Job drawing, mm, ordinate dimensions from the low corner. One solid piece. Coordinates: 2 decimals unless noted, no trailing zeros. Loops run counter-clockwise (first coordinate to the right, second up) from the corner with the lowest first, then second, coordinate; pieces in that order, holes last. Notation, with made-up numbers: (-37.75, -19) - (-27.75, -19) arc R23 cw to (-27.75, 18) - close; hole circle Ø1 at (32.25, -25.75). An arc over 180 degrees is marked (long way). Use a Markdown table: item, result. Add a question column.
1. Wall check: probe 1 along Y at (x, z) = (6.75, 352.7); probe 2 along Z at (x, y) = (18.25, 10); probe 3 along Z at (x, y) = (1.5, 14.25). Give the ranges that are in metal, low to high. Write a range as [from, to].
2. Drop flat-ended pins along their axis: pin 1 (1.5 mm diameter, centred on y = 4, z = 226, fed in from -X); pin 2 (4 mm diameter, centred on y = 12.7, z = 352.7, fed in from -X). Give the stop position or say it passes through.
3. Band-saw the part on B-B, the plane z = 352.7. Give the cut face in (x, y), plus the area to 3 significant figures.
4. Band-saw the part on A-A, the plane y = 12.7. Give the cut face in (x, z), plus the area to 3 significant figures.
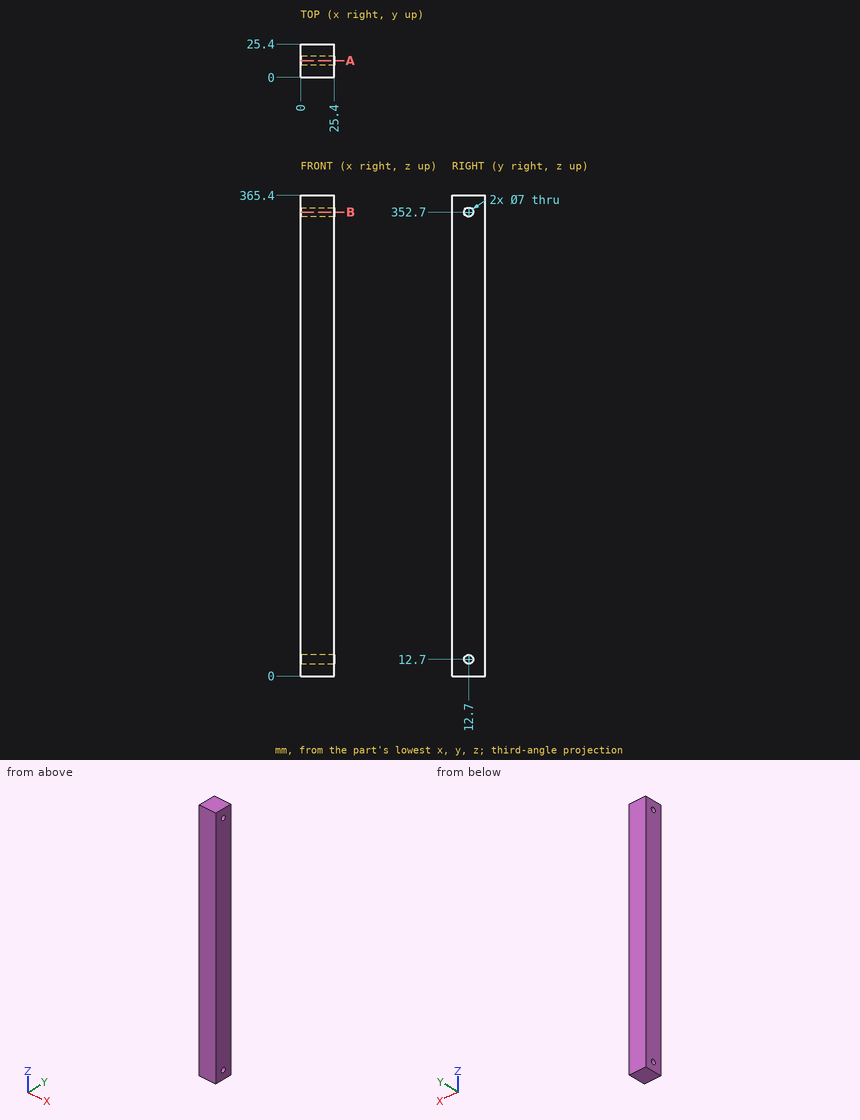
Geometry check:
| question | item | result |
|---|---|---|
| 1 | probe 1 | y = [0, 9.2], [16.2, 25.4] |
| 1 | probe 2 | z = [0, 10.47], [14.93, 350.47], [354.93, 365.4] |
| 1 | probe 3 | z = [0, 9.56], [15.84, 349.56], [355.84, 365.4] |
| 2 | pin 1 | stops at x = 0 |
| 2 | pin 2 | passes through |
| 3 | outline | (0, 0) - (25.4, 0) - (25.4, 9.2) - (0, 9.2) - close; (0, 16.2) - (25.4, 16.2) - (25.4, 25.4) - (0, 25.4) - close |
| 3 | area | 467 mm^2 |
| 4 | outline | (0, 0) - (25.4, 0) - (25.4, 9.2) - (0, 9.2) - close; (0, 16.2) - (25.4, 16.2) - (25.4, 349.2) - (0, 349.2) - close; (0, 356.2) - (25.4, 356.2) - (25.4, 365.4) - (0, 365.4) - close |
| 4 | area | 8,930 mm^2 |
